CAD build for the part. Positions are in the model's coordinates, mm. A direction names the side the tool comes from. Give positions to 0.01 mm unless a question says otherwise; leave off trailing zeros. Order: outer loops, then holes, each group sorted by start corner. A loop starts at its lowest first (then second) coordinate and runs counter-clockwise, first axis right, second up.
Autodesk Inventor part; units mm, degrees
ref_plane "YZ Plane" through (0, 0, 0) normal (1, 0, 0) x (0, 1, 0)
ref_plane "XZ Plane" through (0, 0, 0) normal (0, 1, 0) x (-1, 0, 0)
ref_plane "XY Plane" through (0, 0, 0) normal (0, 0, 1) x (1, 0, 0)
sketch "Sketch1" plane through (0, 0, 0) normal (0, 0, 1) x (1, 0, 0)
  line L0 (0, 0) -> (25.4, 0)
  line L1 (25.4, 0) -> (25.4, 500)
  line L2 (0, 500) -> (25.4, 500)
  line L3 (0, 0) -> (0, 500)
  line L4 (23.8125, 0) -> (23.8125, 500)
  line L5 (1.5875, 0) -> (1.5875, 500)
  line L6 (25.4, 50) -> (0, 50)
  line L7 (0, 50) -> (0, -250)
  line L8 (0, -250) -> (25.4, -250)
  line L9 (25.4, -250) -> (25.4, 50)
  dimension "d0" = 50
  dimension "d1" = 300
extrude "Extrusion1" add sketch "Sketch1" along normal blind 25.4 contours L3 L6 L5 L0 | L0 L9 L8 L7 | L5 L6 L4 L0 | L4 L6 L1 L0
sketch "Sketch2" plane through (0, 50, 0) normal (0, 1, 0) x (1, 0, 0)
  line L0 (23.8125, -1.5875) -> (1.5875, -1.5875)
  line L1 (1.5875, -1.5875) -> (1.5875, -23.8125)
  line L2 (1.5875, -23.8125) -> (23.8125, -23.8125)
  line L3 (23.8125, -23.8125) -> (23.8125, -1.5875)
  line L4 (23.8125, 23.8125) -> (23.8125, 1.5875)
  line L5 (1.5875, 1.5875) -> (1.5875, 23.8125)
  line L6 (25.4, -25.4) -> (0, -25.4)
  point P0 (0, 0)
  dimension "d4" = 22.225
  dimension "d5" = 1.5875
extrude "Extrusion2" cut sketch "Sketch2" against normal up to next
sketch "Sketch3" plane through (0, 0, 25.4) normal (0, 0, 1) x (1, 0, 0)
  circle A0 centre (12.7, 10) radius 7.5
  line L0 (25.4, -250) -> (25.4, 50)
  line L1 (0, 0) -> (25.4, 0)
  line L2 (0, 0) -> (25.4, 0)
  line L3 (23.8125, 15.05) -> (1.5875, 15.05)
  dimension "d8" = 15
  dimension "d9" = 12.7
  dimension "d10" = 10
extrude "Extrusion3" cut sketch "Sketch3" against normal up to next
sketch "Sketch4" plane through (1.5875, 50, 1.5875) normal (0, 0, 1) x (1, 0, 0)
  circle A0 centre (11.1125, -40) radius 7.5
  circle A1 centre (11.1125, -40) radius 4.5
  point P0 (-1.5875, -50)
  dimension "d13" = 9
extrude "Extrusion4" cut sketch "Sketch4" against normal up to next contours A1
properties part number "CounterWeight"
1. Saw through at C-C on y = 10. Give the cut face in (x, z).
2. Saw through at D-D on y = -196. Give the cut face in (x, z), plus the area to 3 significant figures.
3. Mould opens along Z. For faces 1 (the flat face through (13, -98, 25.4)), 2 (the flat face through (13, -98, 0)), 3 (the cylindrical face through (16.992, 11.352, 0.805)), 4 (the flat face through (13, -98, 23.812)) say: released by +Z, released by -Z, zero draft, split by the parting line, or undercut.
4. Saw through at A-A on z = 20. Give the cut face in (x, y).
5. 3-axis set-ups, long thin cutter, end or side, ignore diameter. For faces 5 (the flat face through (1, -250, 13)), 6 (the cylindrical face through (11.07, 2.68, 24.62)), 7 (the flat face through (13, -98, 1.588)): which of +Z, -Z, +X, -X, +Y, -Y reach the whole face in a straight line?
6. Saw through at B-B on x = 12.7. Give the cut face in (y, z), plus the area to 3 significant figures.
7. Wall check: line 1 (X direction, y = 10, z = 24.65); line 2 (Z direction, x = 16.5, y = -204); line 3 (Y direction, x = 12.7, z = 24.45). Give the ranges that are in metal, low to high.
8. Pin check, flat tip, straight feed: P1, Ø12, axis at x = 14.5, z = 16, coming from the -Y side. Stop position of the tip, or through.
Reported:
1. outline: (0, 0) - (8.2, 0) - (8.2, 1.59) - (1.59, 1.59) - (1.59, 23.81) - (5.2, 23.81) - (5.2, 25.4) - (0, 25.4) - close; (17.2, 0) - (25.4, 0) - (25.4, 25.4) - (20.2, 25.4) - (20.2, 23.81) - (23.81, 23.81) - (23.81, 1.59) - (17.2, 1.59) - close
2. outline: (0, 0) - (25.4, 0) - (25.4, 25.4) - (0, 25.4) - close; hole (1.59, 1.59) - (23.81, 1.59) - (23.81, 23.81) - (1.59, 23.81) - close
2. area: 151 mm2
3. face 1: released by +Z
3. face 2: released by -Z
3. face 3: zero draft
3. face 4: undercut
4. outline: (0, -250) - (1.59, -250) - (1.59, 50) - (0, 50) - close; (23.81, -250) - (25.4, -250) - (25.4, 50) - (23.81, 50) - close
5. face 5: +Z, -Z, +X, -X, -Y
5. face 6: +Z
5. face 7: +Y, -Y
6. outline: (-250, 0) - (5.5, 0) - (5.5, 1.59) - (-250, 1.59) - close; (-250, 23.81) - (2.5, 23.81) - (2.5, 25.4) - (-250, 25.4) - close; (14.5, 0) - (50, 0) - (50, 1.59) - (14.5, 1.59) - close; (17.5, 23.81) - (50, 23.81) - (50, 25.4) - (17.5, 25.4) - close
6. area: 914 mm2
7. line 1: x = 0 to 5.2, 20.2 to 25.4
7. line 2: z = 0 to 1.59, 23.81 to 25.4
7. line 3: y = -250 to 2.5, 17.5 to 50
8. P1: passes through
